Can you work these out from the drawing? Everything is in mm from the part's minimum corner. Round coordinates to 2 decimals unless told otherwise and drop trailing zeros. Order: outer loops, then holes, each group sorted by start corner. A loop starts at its lowest first (then second) coordinate and runs counter-clockwise, first axis right, second up. Notation, with made-up numbers: (-29, 19.5) -> (-7, 19.5) arc R11 cw to (-7, 25.5) -> close; hole circle Ø10 at (-8, 6). An arc over 180 degrees is marked (long way). One line per item, written item: value.
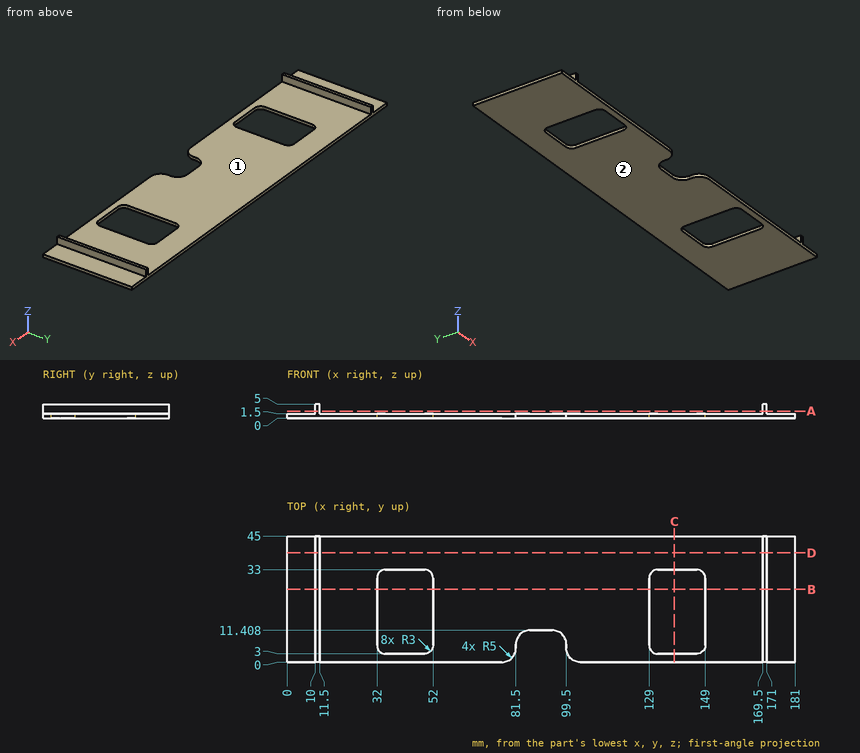
Q1. We'd pull the mould along X, two halves only. Please class the marked faces 1 and 2: released by +X, released by -X, zero draft, split by the parting line, or undercut.
Answers below:
face 1: undercut
face 2: zero draft
Q2. Will these pins go through, and if not, where does the flat tip stop? pin 1 Ø2 at (y, z) = (29.5, 4.5) entering from +X; pin 2 Ø1.1 at (y, z) = (5.5, 0.5) entering from -X; pin 3 Ø1.5 at (x, y) = (61, 28.5) entering from +Z; pin 4 Ø1 at (y, z) = (28.5, 4) entering from -X.
Answers below:
pin 1: x = 171
pin 2: x = 0
pin 3: z = 1.5
pin 4: x = 10
Q3. Please list where these lines run through material, in increasing order: line 1 along X through (y, z) = (13, 0.95); line 2 along X through (y, z) = (42, 4.7); line 3 along X through (y, z) = (4.5, 1.45) (1 decimal).
Answers below:
line 1: 0 to 32, 52 to 129, 149 to 181
line 2: 10 to 11.5, 169.5 to 171
line 3: 0 to 32.4, 51.6 to 81.5, 99.5 to 129.4, 148.6 to 181
Q4. I want a section at C-C on x = 138. List the corners of the cut face in (y, z) for me, plus the area to 3 significant figures.
Answers below:
outline: (0, 0) -> (3, 0) -> (3, 1.5) -> (0, 1.5) -> close; (33, 0) -> (45, 0) -> (45, 1.5) -> (33, 1.5) -> close
area: 22.5 mm^2
Q5. I want a section at A-A on z = 2.5. List the corners of the cut face in (x, y) for me, plus the area to 3 significant figures.
Answers below:
outline: (10, 0) -> (11.5, 0) -> (11.5, 45) -> (10, 45) -> close; (169.5, 0) -> (171, 0) -> (171, 45) -> (169.5, 45) -> close
area: 135 mm^2
Q6. I want a section at D-D on y = 39. List the corners of the cut face in (x, z) for me.
Answers below:
outline: (0, 0) -> (181, 0) -> (181, 1.5) -> (171, 1.5) -> (171, 5) -> (169.5, 5) -> (169.5, 1.5) -> (11.5, 1.5) -> (11.5, 5) -> (10, 5) -> (10, 1.5) -> (0, 1.5) -> close
Q7. I want a section at B-B on y = 26. List the corners of the cut face in (x, z) for me, plus the area to 3 significant figures.
Answers below:
outline: (0, 0) -> (32, 0) -> (32, 1.5) -> (11.5, 1.5) -> (11.5, 5) -> (10, 5) -> (10, 1.5) -> (0, 1.5) -> close; (52, 0) -> (129, 0) -> (129, 1.5) -> (52, 1.5) -> close; (149, 0) -> (181, 0) -> (181, 1.5) -> (171, 1.5) -> (171, 5) -> (169.5, 5) -> (169.5, 1.5) -> (149, 1.5) -> close
area: 222 mm^2
